Can you work these out from the model? Positions are in its coordinate system, mm. A direction names the side the tool comes from. Round coordinates to 2 decimals unless told otherwise and drop trailing zeros. Write each loop counter-clockwise with the first axis right and the second up, starting at its lowest first coordinate (ties: lowest second). Pieces come first, ordered by that corner, then holes.
Q1. Please list where these lines run through material, in increasing order: line 1 along Z through (x, y) = (0, 7.75); line 2 along Z through (x, y) = (150, 48); line 3 along Y through (x, z) = (44, 1.5).
Q2. If we section it at B-B (z = 18.75): Please give me the cut outline in (x, y).
Q3. We'd pull the mould along X, two halves only. Please class faces 1 (the flat face through (74, 20, 26)), 2 (the cylindrical face through (-9.091, 12.325, 22.293)), 3 (the flat face through (150, 39, 4)): +X half, -X half, draft (parallel to the pull), parting line (faces both ways), or undercut.
Q4. If we section it at D-D (y = 41): Please give me the cut outline in (x, z), plus the area to 3 significant figures.
Q5. If we section it at A-A (x = 25): Please give me the cut outline in (y, z), plus the area to 3 significant figures.
Q6. I'm going to push flat-ended pins straight in: pin 1 Ø8 at (y, z) = (42.5, 11.5) entering from -X; pin 2 Ø10 at (x, z) = (120.5, 4.5) entering from -Y; pin 3 Ø8 at (y, z) = (18, 11.5) entering from +X. Where does each tip first touch, or does it pass through?
Q7. For faces 4 (the flat face through (141, 39, 13)), 5 (the flat face through (24, 25, 10)), 6 (the flat face through (-13, 12, 6)), 7 (the cylindrical face through (160.063, 28.472, 16.169)), which set-ups out of +Z, -Z, +X, -X, +Y, -Y let a thin tool reach every point of the face, with its end or its side?
Q8. If we section it at C-C (y = 21): Please give me the cut outline in (x, z), plus the area to 3 significant figures.
Autodesk Inventor part; units mm, degrees
ref_plane "YZ Plane" through (0, 0, 0) normal (1, 0, 0) x (0, 1, 0)
ref_plane "XZ Plane" through (0, 0, 0) normal (0, 1, 0) x (-1, 0, 0)
ref_plane "XY Plane" through (0, 0, 0) normal (0, 0, 1) x (1, 0, 0)
sketch "Sketch1" plane through (0, 0, 0) normal (0, 0, 1) x (1, 0, 0)
  line L0 (0, 0) -> (60, 0)
  arc A0 (60, 0) -> (101.2397, 16.8131) centre (60, 58.9835) ccw
  arc A1 (125, 26.5) -> (101.2397, 16.8131) centre (125, -7.4835) ccw
  line L1 (125, 26.5) -> (150, 26.5)
  line L2 (150, 26.5) -> (150, 51.5)
  line L3 (150, 51.5) -> (125, 51.5)
  arc A2 (125, 51.5) -> (83.7603, 34.6869) centre (125, -7.4835) ccw
  arc A3 (60, 25) -> (83.7603, 34.6869) centre (60, 58.9835) ccw
  line L4 (60, 25) -> (0, 25)
  line L5 (0, 25) -> (0, 0)
  dimension "d0" = 25
  dimension "d1" = 60
  dimension "d2" = 25
  dimension "d3" = 150
  dimension "d4" = 1.5
extrude "Extrusion1" add sketch "Sketch1" along normal blind 26
sketch "Sketch2" plane through (125, 26.5, 0) normal (0, -1, 0) x (1, 0, 0)
  line L0 (25, 0) -> (25, 26)
  circle A0 centre (25, 13) radius 13
  point P0 (-125, 0)
extrude "Extrusion2" add sketch "Sketch2" against normal up to surface (25 mm away)
sketch "Sketch3" plane through (0, 0, 0) normal (0, -1, 0) x (1, 0, 0)
  line L0 (0, 0) -> (0, 26)
  circle A0 centre (0, 13) radius 13
  line L1 (0, 0) -> (-13, 0)
  line L2 (-13, 0) -> (-13, 13)
extrude "Extrusion3" add sketch "Sketch3" against normal up to surface (25 mm away)
sketch "Sketch4" plane through (125, 26.5, 0) normal (0, -1, 0) x (1, 0, 0)
  line L0 (0, 0) -> (25, 0)
  arc A0 (25, 0) -> (25, 26) centre (25, 13) ccw
  line L1 (25, 0) -> (38, 0)
  line L2 (38, 0) -> (38, 13)
  point P0 (-125, 0)
extrude "Extrusion4" add sketch "Sketch4" against normal up to surface (25 mm away)
sketch "Sketch5" plane through (60, 0, 0) normal (0, -1, 0) x (1, 0, 0)
  arc A0 (-60, 26) -> (-73, 13) centre (-60, 13) ccw
  circle A1 centre (-60, 13) radius 4.1
  point P0 (-60, 0)
  dimension "d13" = 8.2
extrude "Extrusion5" cut sketch "Sketch5" against normal through all
sketch "Sketch6" plane through (60, 0, 0) normal (0, -1, 0) x (1, 0, 0)
  arc A0 (-60, 26) -> (-73, 13) centre (-60, 13) ccw
  line L0 (-73, 13) -> (-73, 0)
  line L1 (-60, 13) -> (-35, 13)
  circle A1 centre (-35, 13) radius 1.5
  point P0 (-60, 0)
  dimension "d17" = 3
  dimension "d19" = 25
extrude "Extrusion6" cut sketch "Sketch6" against normal through all
sketch "Sketch7" plane through (125, 26.5, 0) normal (0, -1, 0) x (1, 0, 0)
  arc A0 (38, 13) -> (25, 26) centre (25, 13) ccw
  circle A1 centre (25, 13) radius 10.5 construction
  circle A2 centre (25, 13) radius 7.5 construction
  line L0 (21.2721, 22) -> (28.7279, 22)
  line L1 (28.7279, 22) -> (34, 16.7279)
  line L2 (34, 16.7279) -> (34, 9.2721)
  line L3 (34, 9.2721) -> (28.7279, 4)
  line L4 (28.7279, 4) -> (21.2721, 4)
  line L5 (21.2721, 4) -> (16, 9.2721)
  line L6 (16, 9.2721) -> (16, 16.7279)
  line L7 (16, 16.7279) -> (21.2721, 22)
  point P0 (-125, 0)
  dimension "d22" = 21
  dimension "d24" = 15
  dimension "d25" = 18
extrude "Extrusion7" cut sketch "Sketch7" against normal through all
sketch "Sketch8" plane through (125, 26.5, 0) normal (0, -1, 0) x (1, 0, 0)
  line L0 (16, 16.7279) -> (21.2721, 22)
  line L1 (21.2721, 22) -> (28.7279, 22)
  line L2 (28.7279, 22) -> (34, 16.7279)
  line L3 (34, 16.7279) -> (34, 9.2721)
  line L4 (34, 9.2721) -> (28.7279, 4)
  line L5 (28.7279, 4) -> (21.2721, 4)
  line L6 (21.2721, 4) -> (16, 9.2721)
  line L7 (16, 9.2721) -> (16, 16.7279)
  arc A0 (38, 13) -> (25, 26) centre (25, 13) ccw
  circle A1 centre (25, 13) radius 10.55
  point P0 (-125, 0)
  dimension "d28" = 21.1
extrude "Extrusion8" cut sketch "Sketch8" against normal blind 4
sketch "Sketch9" plane through (125, 51.5, 26) normal (0, 1, 0) x (1, 0, 0)
  line L0 (21.2721, 4) -> (16, 9.2721)
  line L1 (16, 9.2721) -> (16, 16.7279)
  line L2 (16, 16.7279) -> (21.2721, 22)
  line L3 (21.2721, 22) -> (28.7279, 22)
  line L4 (28.7279, 22) -> (34, 16.7279)
  line L5 (34, 16.7279) -> (34, 9.2721)
  line L6 (34, 9.2721) -> (28.7279, 4)
  line L7 (28.7279, 4) -> (21.2721, 4)
  circle A0 centre (25, 13) radius 10.55
  point P0 (-125, 26)
extrude "Extrusion9" cut sketch "Sketch9" against normal blind 4
properties part number "xy forearm"
A:
1. line 1: z = 0 to 8.9, 17.1 to 26
1. line 2: z = 0 to 2.45, 23.55 to 26
1. line 3: y = 0 to 25
2. outline: (-11.66, 0) - (60, 0) arc R58.98 ccw to (101.24, 16.81) arc R33.98 cw to (125, 26.5) - (141.15, 26.5) - (141.15, 30.5) - (143.02, 30.5) - (143.02, 47.5) - (141.15, 47.5) - (141.15, 51.5) - (125, 51.5) arc R58.98 ccw to (83.76, 34.69) arc R33.98 cw to (60, 25) - (-11.66, 25) - close; (156.98, 30.5) - (158.85, 30.5) - (158.85, 26.5) - (161.66, 26.5) - (161.66, 51.5) - (158.85, 51.5) - (158.85, 47.5) - (156.98, 47.5) - close
3. face 1: draft
3. face 2: -X half
3. face 3: undercut
4. outline: (91.41, 0) - (163, 0) - (163, 13) arc R13 ccw to (150, 26) - (91.41, 26) - close; hole (141, 9.27) - (146.27, 4) - (153.73, 4) - (159, 9.27) - (159, 16.73) - (153.73, 22) - (146.27, 22) - (141, 16.73) - close
4. area: 1,560 mm2
5. outline: (0, 0) - (25, 0) - (25, 11.5) - (0, 11.5) - close; (0, 14.5) - (25, 14.5) - (25, 26) - (0, 26) - close
5. area: 575 mm2
6. pin 1: stops at x = 88.06
6. pin 2: stops at y = 25.15
6. pin 3: stops at x = 108.1
7. face 4: +Y, -Y
7. face 5: +Z, -Z, -X, +Y
7. face 6: +Z, -Z, -X, +Y, -Y
7. face 7: -Y
8. outline: (-13, 0) - (106.46, 0) - (106.46, 26) - (0, 26) arc R13 ccw to (-13, 13) - close; hole circle Ø8.2 at (0, 13); hole circle Ø3 at (25, 13)
8. area: 3,010 mm2
